from build123d import *

# Parameters (mm, degrees)
F0_W     = 30
F0_H     = 12
F0_R     = 1.25
F1_DEPTH = 4.8
F2_R     = 1.5
F4_DEPTH = 4.8
F2_W     = 30
F2_H     = 12
F2_R_2   = 2.5
F2_R_3   = 1.25
F5_DEPTH = 3.5
F7_DEPTH = 2.5
F8_SIZE  = 5
F9_SIZE2 = 5
F9_SIZE  = 8


# Not quite as in the source:
# - a fillet or chamfer that OpenCascade refuses, or shapes differently, is made with other operations: its cross-section is extruded or revolved along the edge and cut away or added


with BuildPart() as f1:
    # F0 (on Top) → F1 (new body)
    with BuildSketch(Plane.XY):
        with Locations((0, 0.1359842196)):
            Rectangle(F0_W, F0_H)
        with Locations((-12.8, 0)):
            Circle(F0_R, mode=Mode.SUBTRACT)
        with Locations((12.8, 0)):
            Circle(F0_R, mode=Mode.SUBTRACT)
    extrude(amount=F1_DEPTH)

    # F2 (on face) → F4 (cut, through all)
    with BuildSketch(Plane.XY.offset(4.8)):
        with Locations((-7, -3)):
            Circle(F2_R)
        with Locations((0, 3)):
            Circle(F2_R)
        with Locations((6, -3)):
            Circle(F2_R)
    extrude(amount=-F4_DEPTH, mode=Mode.SUBTRACT)

    # F2 (on face) → F5 (cut)
    with BuildSketch(Plane.XY.offset(4.8)):
        with Locations((0, 0.1359842196)):
            Rectangle(F2_W, F2_H)
        with Locations((-7, -3)):
            Circle(F2_R_2, mode=Mode.SUBTRACT)
        with Locations((-12.8, 0)):
            Circle(F2_R_3, mode=Mode.SUBTRACT)
        with Locations((6, -3)):
            Circle(F2_R_2, mode=Mode.SUBTRACT)
        with Locations((12.8, 0)):
            Circle(F2_R_3, mode=Mode.SUBTRACT)
        with Locations((0, 3)):
            Circle(F2_R_2, mode=Mode.SUBTRACT)
    extrude(amount=-F5_DEPTH, mode=Mode.SUBTRACT)

    # F6: chamfer of 4 x 2 on 3 edges, made by hand


with BuildPart() as f6_tool2:
    # F6_s3 → F6_t4 (revolve)
    with BuildSketch(Plane.XZ.offset(3)):
        Polygon((-2.5, 1.3), (-4.5, 5.3), (-4.5, 1.3), align=None)
    revolve(axis=Axis((-7, -3, 1.3), (0, 0, 1)))

    split(bisect_by=Plane.XZ.offset(5.8640157804), keep=Keep.BOTTOM)

    split(bisect_by=Plane.XY.offset(4.8), keep=Keep.BOTTOM)


with BuildPart() as f1_1:
    add(f1.part)

    # F6_t1: union F6_tool2
    add(f6_tool2.part)


with BuildPart() as f6_tool8:
    # F6_s9 → F6_t10 (revolve)
    with BuildSketch(Plane.XZ.offset(-3)):
        Polygon((4.5, 1.3), (2.5, 5.3), (2.5, 1.3), align=None)
    revolve(axis=Axis((0, 3, 1.3), (0, 0, 1)))

    split(bisect_by=Plane.XZ.offset(-6.1359842196), keep=Keep.TOP)

    split(bisect_by=Plane.XY.offset(4.8), keep=Keep.BOTTOM)


with BuildPart() as f1_2:
    add(f1_1.part)

    # F6_t7: union F6_tool8
    add(f6_tool8.part)


with BuildPart() as f6_tool14:
    # F6_s15 → F6_t16 (revolve)
    with BuildSketch(Plane.XZ.offset(3)):
        Polygon((10.5, 1.3), (8.5, 5.3), (8.5, 1.3), align=None)
    revolve(axis=Axis((6, -3, 1.3), (0, 0, 1)))

    split(bisect_by=Plane.XZ.offset(5.8640157804), keep=Keep.BOTTOM)

    split(bisect_by=Plane.XY.offset(4.8), keep=Keep.BOTTOM)


with BuildPart() as f1_3:
    add(f1_2.part)

    # F6_t13: union F6_tool14
    add(f6_tool14.part)

    # F3 (on face) → F7 (cut)
    with BuildSketch(Plane(origin=(0, 0, 0), x_dir=(1, 0, 0), z_dir=(0, 0, -1))):
        Polygon((-5.2968167059, 5.95), (-8.7031832941, 5.95), (-8.7528263064, 5.8640157804), (-5.2471736936, 5.8640157804), align=None)
        Polygon((7.7528263064, 5.8640157804), (4.2471736936, 5.8640157804), (2.5936334118, 3), (4.2968167059, 0.05), (7.7031832941, 0.05), (9.4063665882, 3), align=None)
        Polygon((-1.7031832941, -5.95), (1.7031832941, -5.95), (3.4063665882, -3), (1.7031832941, -0.05), (-1.7031832941, -0.05), (-3.4063665882, -3), align=None)
        Polygon((-5.2471736936, 5.8640157804), (-8.7528263064, 5.8640157804), (-10.4063665882, 3), (-8.7031832941, 0.05), (-5.2968167059, 0.05), (-3.5936334118, 3), align=None)
    extrude(amount=-F7_DEPTH, mode=Mode.SUBTRACT)

    # F8 (call 1 of 4: OpenCascade refuses the feature's edges together)
    f8_edges = [f1_3.edges().sort_by_distance(p)[0] for p in [
        (-15, 6.135984, 0.65),
    ]]
    chamfer(f8_edges, length=F8_SIZE)

    # F8#2 (call 2 of 4)
    f8_2_edges = [f1_3.edges().sort_by_distance(p)[0] for p in [
        (-15, -5.864016, 0.65),
    ]]
    chamfer(f8_2_edges, length=F8_SIZE)

    # F8#3 (call 3 of 4)
    f8_3_edges = [f1_3.edges().sort_by_distance(p)[0] for p in [
        (15, 6.135984, 0.65),
    ]]
    chamfer(f8_3_edges, length=F8_SIZE)

    # F8#4 (call 4 of 4)
    f8_4_edges = [f1_3.edges().sort_by_distance(p)[0] for p in [
        (15, -5.864016, 0.65),
    ]]
    chamfer(f8_4_edges, length=F8_SIZE)

    # F9
    f9_edges = [f1_3.edges().sort_by_distance(p)[0] for p in [
        (10, 6.135984, 0.65),
        (-10, 6.135984, 0.65),
    ]]
    f9_side = f1_3.faces().sort_by_distance((0, 6.135984, 1.172283))[0]
    chamfer(f9_edges, length=F9_SIZE, length2=F9_SIZE2, reference=f9_side)


solid = f1_3.part
Geometry check sheet. Reference: the model listing, model coordinates, mm. A direction names the side the tool comes from. Round coordinates to 2 decimals unless told otherwise and drop trailing zeros. Order: outer loops, then holes, each group sorted by start corner. A loop starts at its lowest first (then second) coordinate and runs counter-clockwise, first axis right, second up. Notation, with made-up numbers: M 36.5,-1.75 L 67.5,-1.75 A13 cw 67.5,17.25 Z; hole C -8.75,73.5 d3. An arc over 180 degrees is marked long. Write each question's results on one line, items separated by ' | '. Start each with the question number.
1. Cross-section at C-C on x = 0. Record the boundary of the cut face in (y, z).
2. Cross-section at A-A on x = -12.8. Record the boundary of the cut face in (y, z).
3. Cross-section at D-D on x = 6. Record the boundary of the cut face in (y, z), plus the area to 3 significant figures.
4. Set-up check for faces 1 (the face through (-4.4, -4.4, 1.2)), 2 (the face through (-15, 0, 1)), 3 (the face through (-6, 2, 1.3)), 4 (the face through (-7, -0.05, 1)): record each of +Z, -Z, +X, -X, +Y, -Y from which the full face is reachable in a straight line by a thin tool's end or side.
5. Go/stop test with flat-tipped pins: P1, Ø1.7, axis at x = -7, y = -4, coming from the -Z side; P2, Ø0.8, axis at x = 7, z = 1.5, coming from the -Y side; P3, Ø2, axis at x = 4, z = 2, coming from the +Y side. Record where each tip stops, or that it passes through.
6. Material ranges on L1, parallel to Z at x = -5.75, y = 4; L2, parallel to X at y = -2.5, z = 4.5; L3, parallel to Y at x = -12, z = 0.8, recorded low to high. Write a range as from..to.
7. Cross-section at B-B on z = 0.45. Give the number of separate pieces and of enclosed holes in the cut face, plus the area to 3 significant figures.
8. Draft check along Y on faces 5 (the face through (-9, -3, 2.5)), 6 (the face through (-7.849, 4.343, 0.775)), 7 (the face through (-12.465, -3.399, 0.766)). Enter one of: pulls with the +Y half, pulls with the -Y half, needs draft (parallel to the pull), parting line crosses it, or undercut.
Resolved:
1) outline: M -5.86,0 L 0.05,0 L 0.05,2.5 L 1.5,2.5 L 1.5,4.8 L 0.25,4.8 L -1.5,1.3 L -5.86,1.3 Z; M 4.5,2.5 L 5.95,2.5 L 5.95,0 L 6.14,0 L 6.14,4.03 L 5.75,4.8 L 4.5,4.8 Z
2) outline: M -3.06,0 L -1.25,0 L -1.25,1.3 L -3.06,1.3 Z; M 1.25,0 L 2.83,0 L 2.83,1.3 L 1.25,1.3 Z
3) outline: M -5.86,2.5 L -4.5,2.5 L -4.5,4.8 L -5.75,4.8 L -5.86,4.57 Z; M -1.5,2.5 L -0.05,2.5 L -0.05,0 L 4.91,0 L 4.91,1.3 L 1.5,1.3 L -0.25,4.8 L -1.5,4.8 Z | area: 15.3 mm2
4) face 1: -Z | face 2: +Z, -Z, -X, +Y, -Y | face 3: +Z | face 4: -Z, -Y
5) P1: z = 2.5 | P2: y = -0.05 | P3: y = 5.83
6) L1: 0..1.3 | L2: -9.86..-8.41, -5.59..-4.14, 3.14..4.59, 7.41..8.86 | L3: -3.86..-0.96, 0.96..3.07
7) separate pieces: 1 | enclosed holes: 3 | area: 182 mm2
8) face 5: undercut | face 6: pulls with the +Y half | face 7: pulls with the -Y half
